```python
from build123d import *

# Parameters (mm, degrees)
BOSS_EXTRUDE1_DEPTH = 17
BOSS_EXTRUDE2_DEPTH = 2
BOSS_EXTRUDE3_DEPTH = 2
SKETCH6_R           = 2
CUT_EXTRUDE1_DEPTH  = 10
CUT_EXTRUDE2_DEPTH  = 4
CUT_EXTRUDE3_DEPTH  = 100
CUT_EXTRUDE4_DEPTH  = 4


with BuildPart() as part:
    # Sketch1 → Boss-Extrude1 (new body)
    with BuildSketch(Plane(origin=(0, 0, 0), x_dir=(1, 0, 0), z_dir=(0, 1, 0))):
        Polygon((-7.978390595, -3.663628582), (12.021609405, -3.663628582), (12.021609405, 31.336371418), (28.021609405, 31.336371418), (28.021609405, 27.336371418), (15.021609405, 27.336371418), (15.021609405, 18.231970095), (15.021609405, -16.663628582), (-10.978390595, -16.663628582), (-10.978390595, 22.152823879), (-10.978390595, 27.336371418), (-23.978390595, 27.336371418), (-23.978390595, 31.336371418), (-7.978390595, 31.336371418), align=None)
    extrude(amount=BOSS_EXTRUDE1_DEPTH)

    # Sketch4 → Boss-Extrude2 (add)
    with BuildSketch(Plane(origin=(0, 17, 0), x_dir=(1, 0, 0), z_dir=(0, 1, 0))):
        Polygon((-23.978390595, 27.336371418), (-10.978390595, 14.336371418), (-10.978390595, 27.336371418), align=None)
        Polygon((28.021609405, 27.336371418), (15.021609405, 14.336371418), (15.021609405, 27.336371418), align=None)
    extrude(amount=-BOSS_EXTRUDE2_DEPTH)

    # Sketch5 → Boss-Extrude3 (add)
    with BuildSketch(Plane.XZ):
        Polygon((-23.978390595, -27.336371418), (-10.978390595, -14.336371418), (-10.978390595, -27.336371418), align=None)
        Polygon((15.021609405, -14.336371418), (28.021609405, -27.336371418), (15.021609405, -27.336371418), align=None)
    extrude(amount=-BOSS_EXTRUDE3_DEPTH)

    # Sketch6 → Cut-Extrude1 (cut)
    with BuildSketch(Plane(origin=(0, 0, -31.336371418), x_dir=(-1, 0, 0), z_dir=(0, 0, -1))):
        with Locations((-22.021609405, 8.5)):
            Circle(SKETCH6_R)
        with Locations((17.978390595, 8.5)):
            Circle(SKETCH6_R)
    extrude(amount=-CUT_EXTRUDE1_DEPTH, mode=Mode.SUBTRACT)

    # Sketch7 → Cut-Extrude2 (cut)
    with BuildSketch(Plane(origin=(-7.978390595, 0, 0), x_dir=(0, 0, -1), z_dir=(1, 0, 0))):
        with BuildLine():
            Line((6.660260068, 17), (-15.113860184, 17))
            ThreePointArc((-15.113860184, 17), (-9.316147205, 8.548897323), (-3.663628582, 0))
            Line((-3.663628582, 0), (9.59929213, 0))
            Line((9.59929213, 0), (6.660260068, 17))
        make_face()
    extrude(amount=CUT_EXTRUDE2_DEPTH, mode=Mode.SUBTRACT)

    # Sketch8 → Cut-Extrude3 (cut)
    with BuildSketch(Plane.ZY.offset(10.978390595)):
        with BuildLine():
            Line((21.615286826, 19.275621448), (46.650832109, 12.975800719))
            Line((46.650832109, 12.975800719), (28.995853608, -26.911994427))
            Line((28.995853608, -26.911994427), (-0.690246805, -14.377221046))
            ThreePointArc((-0.690246805, -14.377221046), (10.177476822, 2.638130465), (21.615286826, 19.275621448))
        make_face()
    extrude(amount=-CUT_EXTRUDE3_DEPTH, mode=Mode.SUBTRACT)

    # Sketch9 → Cut-Extrude4 (cut)
    with BuildSketch(Plane.ZY.offset(-12.021609405)):
        with BuildLine():
            Line((-11.188223811, 17), (-11.188223811, 0))
            Line((-11.188223811, 0), (3.663628582, 0))
            ThreePointArc((3.663628582, 0), (9.316147205, 8.548897323), (15.113860184, 17))
            Line((15.113860184, 17), (-11.188223811, 17))
        make_face()
    extrude(amount=CUT_EXTRUDE4_DEPTH, mode=Mode.SUBTRACT)


solid = part.part
```
Geometry: final body of the model. Coordinates: model frame, mm. A direction names the side the tool comes from. Round coordinates to 2 decimals unless told otherwise and drop trailing zeros. Loops run counter-clockwise (first coordinate to the right, second up) from the corner with the lowest first, then second, coordinate; pieces in that order, holes last. Notation, with made-up numbers: (7.5, 18) -> (33.5, 18) arc R26 cw to (33.5, 48) -> close; hole circle Ø5 at (78, 80). An arc over 180 degrees is marked (long way). Use one line per item in the form item = value. Start each with the question number.
1) Section C-C on z = -8. Output: boundary loops of the cut face in (x, y), then the cut area to 3 significant figures.
2) Line query: L1, parallel to Y at x = 19.5, z = -24; L2, parallel to X at y = 13.5, z = -15.5; L3, parallel to X at y = 1.25, z = -28. Output: solid intervals per line, ascending.
3) Draft query along Y for faces 5 (the cylindrical face through (10.05, 8.43, 9.236)), 6 (the flat face through (-17.57, 0.99, -20.93)), 7 (the flat face through (19, 15, -24)). Return one class per face: released by +Y, released by -Y, zero draft, split by the parting line, or undercut.
4) First-contact query: P1, Ø5, axis at y = 7, z = 2.5, coming from the +X side; P2, Ø6, axis at x = -1, y = 2, coming from the -Z side; P3, Ø10, axis at x = -16.5, y = 5, coming from the +Z side. Flat tips, straight axial feed; report the tip coordinate or a pass-through.
5) Section A-A on z = -28. Output: boundary loops of the cut face in (x, y), then the cut area to 3 significant figures.
6) Section B-B on y = 7.5. Output: boundary loops of the cut face in (x, z), then the cut area to 3 significant figures.
7) Section D-D on x = -17. Output: boundary loops of the cut face in (y, z), then the cut area to 3 significant figures.
8) Access query for faces 1 (the flat face through (-10.978, 8, -6)), 2 (the flat face through (19, 2, -24)), 3 (the flat face through (2, 8, 3.664)), 4 (the flat face through (8.022, 11, 8)). Directions: +Z, -Z, +X, -X, +Y, -Y. A direction counts if a zero-diameter tool reaches every point of the face in a straight line with its end or side. Return the directions, or none.
Response:
q1.outline = (-10.98, 0) -> (-7.98, 0) -> (-7.98, 17) -> (-10.98, 17) -> close; (12.02, 0) -> (15.02, 0) -> (15.02, 17) -> (12.02, 17) -> close
q1.area = 102 mm^2
q2.L1 = 0 to 2, 15 to 17
q2.L2 = -10.98 to -7.98, 12.02 to 15.02
q2.L3 = -23.98 to -7.98, 12.02 to 28.02
q3.face_5 = released by +Y
q3.face_6 = zero draft
q3.face_7 = undercut
q4.P1 = 15.02
q4.P2 = 3.66
q4.P3 = -15.86
q5.outline = (-23.98, 0) -> (-7.98, 0) -> (-7.98, 17) -> (-23.98, 17) -> close; (12.02, 0) -> (28.02, 0) -> (28.02, 17) -> (12.02, 17) -> close; hole circle Ø4 at (-17.98, 8.5); hole circle Ø4 at (22.02, 8.5)
q5.area = 519 mm^2
q6.outline = (-23.98, -31.34) -> (-19.71, -31.34) -> (-19.71, -27.34) -> (-23.98, -27.34) -> close; (-16.25, -31.34) -> (-7.98, -31.34) -> (-7.98, 8.61) -> (-3.98, 8.61) -> (-3.98, 3.66) -> (8.02, 3.66) -> (8.02, 8.61) -> (12.02, 8.61) -> (12.02, -31.34) -> (20.29, -31.34) -> (20.29, -27.34) -> (15.02, -27.34) -> (15.02, 13.43) -> (-10.98, 13.43) -> (-10.98, -27.34) -> (-16.25, -27.34) -> close; (23.75, -31.34) -> (28.02, -31.34) -> (28.02, -27.34) -> (23.75, -27.34) -> close
q6.area = 501 mm^2
q7.outline = (0, -31.34) -> (6.76, -31.34) -> (6.76, -27.34) -> (2, -27.34) -> (2, -20.36) -> (0, -20.36) -> close; (10.24, -31.34) -> (17, -31.34) -> (17, -20.36) -> (15, -20.36) -> (15, -27.34) -> (10.24, -27.34) -> close
q7.area = 82.0 mm^2
q8.face_1 = +Z, -X
q8.face_2 = +Z, +X
q8.face_3 = -Z, +Y, -Y
q8.face_4 = -Z, +Y
